```python
from build123d import *

# Parameters (mm, degrees)
SKETCH1_R           = 14.2875
BOSS_EXTRUDE1_DEPTH = 3.175
SKETCH3_R           = 12.7
CUT_EXTRUDE2_DEPTH  = 4.175
SKETCH5_W           = 50.8
SKETCH5_H           = 247.65
CUT_EXTRUDE4_DEPTH  = 4.175
SKETCH6_W           = 127
SKETCH6_H           = 25.4
CUT_EXTRUDE5_DEPTH  = 4.175
BOSS_EXTRUDE2_DEPTH = 3.175
FILLET1_R           = 9.525


with BuildPart() as part:
    # Sketch1 → Boss-Extrude1 (new body)
    with BuildSketch(Plane(origin=(0, 0, 0), x_dir=(0, 0, -1), z_dir=(1, 0, 0))):
        Polygon((-50.8, 25.4), (50.8, 25.4), (369.963359856, -60.119564527), (369.963359856, -337.700549698), (319.163359856, -337.700549698), (319.163359856, -99.099775516), (44.112053123, -25.4), (-44.112053123, -25.4), (-282.997152386, -89.409069432), (-296.145159877, -40.340037456), align=None)
        with Locations((-265.036640144, -58.300549698)):
            Circle(SKETCH1_R, mode=Mode.SUBTRACT)
        Circle(SKETCH1_R, mode=Mode.SUBTRACT)
    extrude(amount=BOSS_EXTRUDE1_DEPTH)

    # Sketch3 → Cut-Extrude2 (cut, through all)
    with BuildSketch(Plane(origin=(3.175, 0, 0), x_dir=(0, 0, -1), z_dir=(1, 0, 0))):
        with Locations((344.563359856, -312.300549698)):
            Circle(SKETCH3_R)
    extrude(amount=-CUT_EXTRUDE2_DEPTH, mode=Mode.SUBTRACT)

    # Sketch5 → Cut-Extrude4 (cut, through all)
    with BuildSketch(Plane(origin=(3.175, 0, 0), x_dir=(0, 0, -1), z_dir=(1, 0, 0))):
        with Locations((344.563359856, -213.875549698)):
            Rectangle(SKETCH5_W, SKETCH5_H)
    extrude(amount=-CUT_EXTRUDE4_DEPTH, mode=Mode.SUBTRACT)

    # Sketch6 → Cut-Extrude5 (cut, through all)
    with BuildSketch(Plane(origin=(3.175, 0, 0), x_dir=(0, 0, -1), z_dir=(1, 0, 0))):
        with Locations((306.463359856, -102.750549698)):
            Rectangle(SKETCH6_W, SKETCH6_H)
    extrude(amount=-CUT_EXTRUDE5_DEPTH, mode=Mode.SUBTRACT)

    # Sketch7 → Boss-Extrude2 (add)
    with BuildSketch(Plane(origin=(3.175, 0, 0), x_dir=(0, 0, -1), z_dir=(1, 0, 0))):
        Polygon((292.079136211, -39.250549698), (369.963359856, -39.250549698), (369.963359856, -60.119564527), align=None)
    extrude(amount=-BOSS_EXTRUDE2_DEPTH)

    # Fillet1
    fillet1_edges = [part.edges().sort_by_distance(p)[0] for p in [
        (1.5875, 25.4, 50.8),
        (1.5875, 25.4, -50.8),
        (1.5875, -25.4, -44.112053123),
        (1.5875, -25.4, 44.112053123),
        (1.5875, -89.409069432, 282.997152386),
        (1.5875, -40.340037456, 296.145159877),
        (1.5875, -90.050549698, -369.963359856),
        (1.5875, -90.050549698, -285.391189333),
        (1.5875, -39.250549698, -292.079136211),
        (1.5875, -39.250549698, -369.963359856),
    ]]
    fillet(fillet1_edges, radius=FILLET1_R)


solid = part.part
```
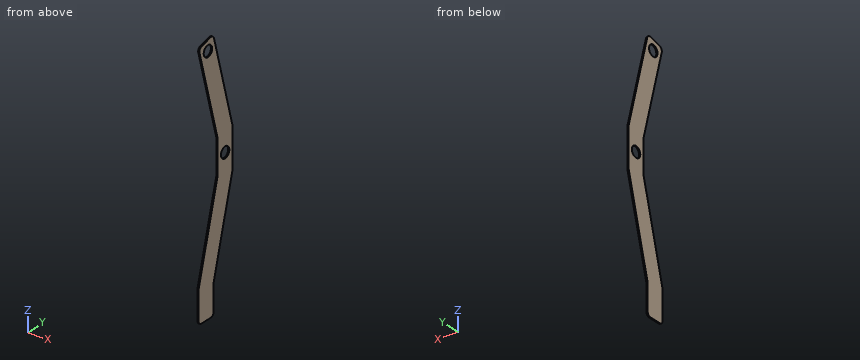
Verification items for the finished model (mm, model axes). Round coordinates to 2 decimals unless told otherwise and drop trailing zeros. Write each loop counter-clockwise with the first axis right and the second up, starting at its lowest first coordinate (ties: lowest second). Pieces come first, ordered by that corner, then holes. Notation, with made-up numbers: (-3, 66.5) -> (38, 66.5) arc R18 cw to (38, 81.5) -> close; hole circle Ø1 at (68.5, 26). An arc over 180 degrees is marked (long way). Write each question's results on one line, items separated by ' | '. Start each with the question number.
1. Cross-section at C-C (x = 0.6). Count the separate pieces of the cut face and the enclosed holes in it, then the cut area to 3 significant figures.
2. Cross-section at D-D (z = 122.5). Enter the section's corners in (x, y) (3 decimals).
3. Material ranges on probe 1 along Y at (x, z) = (2.25, 0); probe 2 along Y at (x, z) = (2.35, -294.5); probe 3 along Y at (x, z) = (0.55, 199.5), recorded low to high. Write a range as from..to.
4. Depth check by flat-ended pin: P1, Ø1.5, axis at x = 0.5, z = -202, coming from the +Y side; P2, Ø1, axis at x = 2, z = 222, coming from the +Y side; P3, Ø23, axis at y = 0, z = 0, coming from the +X side. Enter the tip coordinate at first touch or a pass-through.
5. Cross-section at A-A (z = 0). Enter the section's corners in (x, y) (1 decimal).
6. Cross-section at B-B (y = 0). Enter the section's corners in (x, z) (1 decimal).
Solutions:
1) separate pieces: 1 | enclosed holes: 2 | area: 33,000 mm2
2) outline: (0, -46.404) -> (3.175, -46.404) -> (3.175, 6.188) -> (0, 6.188) -> close
3) probe 1: y = -25.4..-14.29, 14.29..25.4 | probe 2: y = -90.05..-39.25 | probe 3: y = -67.04..-14.44
4) P1: stops at y = -14.91 | P2: stops at y = -20.34 | P3: passes through
5) outline: (0, -25.4) -> (3.2, -25.4) -> (3.2, -14.3) -> (0, -14.3) -> close; (0, 14.3) -> (3.2, 14.3) -> (3.2, 25.4) -> (0, 25.4) -> close
6) outline: (0, -145.6) -> (3.2, -145.6) -> (3.2, -14.3) -> (0, -14.3) -> close; (0, 14.3) -> (3.2, 14.3) -> (3.2, 145.6) -> (0, 145.6) -> close
